```python
from build123d import *

# Parameters (mm, degrees)
BOSS_EXTRUDE1_DEPTH = 14.2875
SKETCH4_R           = 2.159
CUT_EXTRUDE2_DEPTH  = 27.126252203
BOSS_EXTRUDE3_DEPTH = 2.38125


with BuildPart() as part:
    # Sketch1 → Boss-Extrude1 (new body)
    with BuildSketch(Plane.XY):
        with BuildLine():
            Line((-4.7625, 0), (-4.7625, 16.5862))
            ThreePointArc((-4.7625, 16.5862), (0, 21.3487), (4.7625, 16.5862))
            Line((4.7625, 16.5862), (4.7625, 0))
            ThreePointArc((4.7625, 0), (0, -4.7625), (-4.7625, 0))
        make_face()
    extrude(amount=BOSS_EXTRUDE1_DEPTH)

    # Sketch4 → Cut-Extrude2 (cut, through all)
    with BuildSketch(Plane.XY.offset(14.2875)):
        with Locations((0, 16.5862)):
            Circle(SKETCH4_R)
        Circle(SKETCH4_R)
    extrude(amount=-CUT_EXTRUDE2_DEPTH, mode=Mode.SUBTRACT)

    # Sketch5 → Boss-Extrude3 (add)
    with BuildSketch(Plane.XY.offset(14.2875)):
        with BuildLine():
            Line((-4.7625, 4.559746601), (-4.7625, 12.026453399))
            ThreePointArc((-4.7625, 12.026453399), (-3.909869704, 13.43362175), (-2.267857143, 13.329238142))
            ThreePointArc((-2.267857143, 13.329238142), (0, 12.61745), (2.267857143, 13.329238142))
            ThreePointArc((2.267857143, 13.329238142), (3.909869704, 13.43362175), (4.7625, 12.026453399))
            Line((4.7625, 12.026453399), (4.7625, 4.559746601))
            ThreePointArc((4.7625, 4.559746601), (3.909869704, 3.15257825), (2.267857143, 3.256961858))
            ThreePointArc((2.267857143, 3.256961858), (0, 3.96875), (-2.267857143, 3.256961858))
            ThreePointArc((-2.267857143, 3.256961858), (-3.909869704, 3.15257825), (-4.7625, 4.559746601))
        make_face()
    extrude(amount=BOSS_EXTRUDE3_DEPTH)


solid = part.part
```
Geometry check sheet. Reference: the model listing, model coordinates, mm. A direction names the side the tool comes from. Coordinates: 2 decimals unless noted, no trailing zeros. Write each loop counter-clockwise with the first axis right and the second up, starting at its lowest first coordinate (ties: lowest second). Pieces come first, ordered by that corner, then holes. Notation, with made-up numbers: M 22.25,-23.5 L 65.25,-23.5 A30 ccw 65.25,7.5 Z; hole C -40,78 d7. An arc over 180 degrees is marked long. One line per item, written item: value. Start each with the question number.
(1) Sectioned sample at D-D, the plane x = 3.5. Enter the section's corners in (y, z), and give its area (3 significant figures).
(2) Scan lines: line 1 along Y through (x, z) = (0, 8); line 2 along Y through (x, z) = (1.25, 7.5); line 3 along X through (y, z) = (16.5, 10.5). Record each from-to range of solid material in increasing order. Write a range as [from, to].
(3) Release check for a two-part mould opening along X. For faces 4 (the face through (0.03, 3.97, 15.46)), 5 (the face through (-4.762, 8, 8)), 6 (the face through (-0.105, 21.348, 7.044)) record: released by +X, released by -X, zero draft, split by the parting line, or undercut.
(4) Depth check by flat-ended pin: pin 1 (8 mm diameter, centred on y = -1.5, z = 4.5, fed in from -X); pin 2 (5 mm diameter, centred on x = 0, y = 16.59, fed in from +Z). Enter the tip coordinate at first touch or a pass-through.
(5) Sectioned sample at B-B, the plane y = 0.5. Enter the section's corners in (x, z), and give its area (3 significant figures).
(6) Tool access check on faces 1 (the face through (3.931, 3.164, 15.461)), 2 (the face through (3.888, 13.445, 15.461)), 3 (the face through (0, 8, 16.669)). Record the directions out of +Z, -Z, +X, -X, +Y, -Y that give a thin tool (end or side, any length) a straight path to the whole face; none if there is none.
(7) Sectioned sample at C-C, the plane z = 11.75. Enter the section's corners in (x, y) (1 decimal), and give its area (3 significant figures).
(8) Sectioned sample at A-A, the plane x = 0. Enter the section's corners in (y, z), and give its area (3 significant figures).
Filled sheet:
1. outline: M -3.23,0 L 19.82,0 L 19.82,14.29 L 13.58,14.29 L 13.58,16.67 L 3.01,16.67 L 3.01,14.29 L -3.23,14.29 Z
1. area: 354 mm²
2. line 1: [-4.76, -2.16], [2.16, 14.43], [18.75, 21.35]
2. line 2: [-4.6, -1.76], [1.76, 14.83], [18.35, 21.18]
2. line 3: [-4.76, -2.16], [2.16, 4.76]
3. face 4: undercut
3. face 5: released by -X
3. face 6: split by the parting line
4. pin 1: x = -4.76
4. pin 2: z = 14.29
5. outline: M -4.76,0 L -2.1,0 L -2.1,14.29 L -4.76,14.29 Z; M 2.1,0 L 4.76,0 L 4.76,14.29 L 2.1,14.29 Z
5. area: 76.1 mm²
6. face 1: +Z, -Y
6. face 2: +Z, +Y
6. face 3: +Z, +X, -X, +Y, -Y
7. outline: M -4.8,0 A4.8 ccw 4.8,0 L 4.8,16.6 A4.8 ccw -4.8,16.6 Z; hole C 0,0 d4.3; hole C 0,16.6 d4.3
7. area: 200 mm²
8. outline: M -4.76,0 L -2.16,0 L -2.16,14.29 L -4.76,14.29 Z; M 2.16,0 L 14.43,0 L 14.43,14.29 L 12.62,14.29 L 12.62,16.67 L 3.97,16.67 L 3.97,14.29 L 2.16,14.29 Z; M 18.75,0 L 21.35,0 L 21.35,14.29 L 18.75,14.29 Z
8. area: 270 mm²
